from build123d import *

# Parameters (mm, degrees)
BOSS_EXTRUDE1_DEPTH            = 2
BOSS_EXTRUDE2_DEPTH            = 17.5
BOSS_EXTRUDE2_DEPTH_BACK       = 17.5
SKETCH2_R                      = 1.7500000000000036
SKETCH3_R                      = 2.999999999999994
CUT_EXTRUDE1_DEPTH             = 6.75
CUT_EXTRUDE2_DEPTH             = 2
BOSS_EXTRUDE4_DEPTH            = 3
BOSS_EXTRUDE4_DEPTH_BACK       = 0.5
SKETCH6_R                      = 1.7500000000000036
CUT_EXTRUDE3_DEPTH             = 77.9415362466854
FILLET1_R                      = 1
SKETCH7_W                      = 9
SKETCH7_H                      = 6
CUT_EXTRUDE4_DEPTH             = 2
FILLET2_R                      = 3
FILLET3_R                      = 3
CUT_EXTRUDE5_REACH             = 78.455
SKETCH10_R                     = 2.999999999999994
CUT_EXTRUDE5_DIRECTION_2_REACH = 78.455
BOSS_EXTRUDE6_DEPTH            = 1
BOSS_EXTRUDE6_DEPTH_BACK       = 1
SKETCH11_R                     = 0.7499999999999987
FILLET5_R                      = 1.5


# Some blends are built 0.0001 mm under size
with BuildPart() as part:
    # Sketch1 → Boss-Extrude1 (new body)
    with BuildSketch(Plane(origin=(0, 0, 0), x_dir=(1, 0, 0), z_dir=(0, 1, 0))):
        with BuildLine():
            Line((-17.499999999999993, -42), (17.499999999999993, -42))
            ThreePointArc((17.499999999999993, -42), (45.5, 1.01e-14), (17.499999999999975, 42.00000000000001))
            Line((17.499999999999975, 42.00000000000001), (-17.499999999999975, 42.00000000000001))
            ThreePointArc((-17.499999999999975, 42.00000000000001), (-45.5, 5.57e-15), (-17.499999999999993, -42))
        make_face()
    extrude(amount=BOSS_EXTRUDE1_DEPTH)

    # Sketch2 → Boss-Extrude2 (add, two sides: drawn at the far end of the back side and taken through both)
    with BuildSketch(Plane(origin=(0, 0, 0), x_dir=(0, 0, -1), z_dir=(1, 0, 0)).offset(-BOSS_EXTRUDE2_DEPTH_BACK)):
        with BuildLine():
            Line((-42, 0), (-42.171572875253815, 0))
            ThreePointArc((-42.171572875253815, 0), (-48.00000000000001, 1.0000000000000004), (-42.171572875253815, 2))
            Line((-42.171572875253815, 2), (-42, 2))
            Line((-42, 2), (-42, 1))
            Line((-42, 1), (-42, 0))
        make_face()
        with Locations((-45.00000000000001, 1)):
            Circle(SKETCH2_R, mode=Mode.SUBTRACT)
    extrude(amount=BOSS_EXTRUDE2_DEPTH + BOSS_EXTRUDE2_DEPTH_BACK)

    # Sketch3 → Cut-Extrude1 (cut)
    with BuildSketch(Plane(origin=(3.5, 0, 0), x_dir=(0, 0, -1), z_dir=(1, 0, 0))):
        with Locations((-45.00000000000001, 1)):
            Circle(SKETCH3_R)
    cut_extrude1 = extrude(amount=CUT_EXTRUDE1_DEPTH, mode=Mode.SUBTRACT)

    # Mirror1: Cut-Extrude1 across plane
    add(cut_extrude1.mirror(Plane(origin=(0, 0, 0), x_dir=(0, 0, 1), z_dir=(1, 0, 0))), mode=Mode.SUBTRACT)

    # Sketch4 → Cut-Extrude2 (cut)
    with BuildSketch(Plane(origin=(0, 2, 0), x_dir=(1, 0, 0), z_dir=(0, 1, 0))):
        Polygon((0.7499999999999764, 42.00000000000001), (21.249999999999982, 42.00000000000001), (21.24999999999998, 32.75000000000001), (0.7499999999999775, 32.75000000000001), (0.7499999999999781, 35.00000000000001), (-17.50000000000002, 35.00000000000001), (-17.50000000000002, 42.00000000000001), align=None)
    extrude(amount=-CUT_EXTRUDE2_DEPTH, mode=Mode.SUBTRACT)

    # Sketch5 → Boss-Extrude4 (add, two sides: drawn at the far end of the back side and taken through both)
    with BuildSketch(Plane(origin=(-17.50000000000002, 0, 0), x_dir=(0, 0, -1), z_dir=(1, 0, 0)).offset(-BOSS_EXTRUDE4_DEPTH_BACK)):
        with BuildLine():
            Line((35.00000000000001, 1), (35.00000000000001, 2))
            Line((35.00000000000001, 2), (38.171572875253815, 2))
            ThreePointArc((38.171572875253815, 2), (44.00000000000001, 1), (38.171572875253815, 0))
            Line((38.171572875253815, 0), (35.00000000000001, 0))
            Line((35.00000000000001, 0), (35.00000000000001, 1))
        make_face()
    extrude(amount=BOSS_EXTRUDE4_DEPTH + BOSS_EXTRUDE4_DEPTH_BACK)

    # Sketch6 → Cut-Extrude3 (cut, through all)
    with BuildSketch(Plane(origin=(-14.500000000000023, 0, 0), x_dir=(0, 0, -1), z_dir=(1, 0, 0))):
        with Locations((41.00000000000001, 1)):
            Circle(SKETCH6_R)
    extrude(amount=-CUT_EXTRUDE3_DEPTH, mode=Mode.SUBTRACT)

    # Fillet1
    fillet1_edges = [part.edges().sort_by_distance(p)[0] for p in [
        (-20.23555777714238, 0, -39.563859338365496),
        (-20.23555777714238, 2, -39.563859338365496),
    ]]
    fillet(fillet1_edges, radius=FILLET1_R - 0.0001)  # a hair under: the kernel refuses the full size

    # Sketch7 → Cut-Extrude4 (cut)
    with BuildSketch(Plane(origin=(0, 2, 0), x_dir=(1, 0, 0), z_dir=(0, 1, 0))):
        with Locations((24.749999999999975, 38.00000000000001)):
            Rectangle(SKETCH7_W, SKETCH7_H)
    extrude(amount=-CUT_EXTRUDE4_DEPTH, mode=Mode.SUBTRACT)

    # Fillet2
    # the kernel refuses this fillet: 3 mm, written as the material it adds along each edge
    with BuildSketch(Plane(origin=(-14.500000000000021, 0, -35.00000000000001), x_dir=(0, 0, -1), z_dir=(0, 1, 0))) as fillet2_piece_1:
        with BuildLine():
            CenterArc((FILLET2_R, -FILLET2_R), FILLET2_R, 90, 90)
            Line((0, -FILLET2_R), (0, 0))
            Line((0, 0), (FILLET2_R, 0))
        make_face()
    extrude(amount=2)
    # the kernel refuses this fillet: 3 mm, written as the material it takes off along each edge
    with BuildSketch(Plane(origin=(29.07318352021326, 4.856917413714078, -35.00000000000001), x_dir=(-1, 0, 0), z_dir=(0, -1, 0))) as fillet2_2_piece_1:
        with BuildLine():
            CenterArc((1.1044509783192602, -3), FILLET2_R, 90, 41.154201960072044)
            ThreePointArc((-0.8698124952261921, -0.7411764705882291), (-0.43723324041952694, -0.3678573776648406), (0, 0))
            Line((0, 0), (1.1044509783192602, 0))
        make_face()
    extrude(amount=7.7138348274281565, mode=Mode.SUBTRACT)
    with BuildSketch(Plane(origin=(21.24999999999998, -7.261843774138903, -35.00000000000001), x_dir=(0, 0, 1), z_dir=(0, 1, 0))) as fillet2_2_piece_2:
        with BuildLine():
            CenterArc((3, 2.904737509655561), FILLET2_R, 180, 75.52248781407008)
            Line((0, 2.904737509655561), (0, 0))
            Line((0, 0), (2.25, 0))
        make_face()
    extrude(amount=16.523687548277806, mode=Mode.SUBTRACT)
    with BuildSketch(Plane(origin=(0.7499999999999781, 9.261843774138908, -35.00000000000001), x_dir=(-1, 0, 0), z_dir=(0, -1, 0))) as fillet2_2_piece_3:
        with BuildLine():
            CenterArc((2.9047375096555634, -3), FILLET2_R, 90, 75.5224878140701)
            Line((7.8e-16, -2.25), (0, 0))
            Line((0, 0), (2.9047375096555634, 0))
        make_face()
    extrude(amount=16.523687548277817, mode=Mode.SUBTRACT)

    # Fillet3
    fillet3_edges = [part.edges().sort_by_distance(p)[0] for p in [
        (21.24999999999998, 1, -32.75000000000001),
        (0.7499999999999775, 1, -32.75000000000001),
    ]]
    fillet(fillet3_edges, radius=FILLET3_R)

    # Cut-Extrude5: up to this face of the body (flat: up to its plane)
    cut_extrude5_end = Plane(part.part.faces().sort_by_distance((-10.25, 1, 42.084852814))[0])
    # Sketch10 → Cut-Extrude5 (cut, up to the picked face)
    with BuildSketch(Plane.ZY.offset(13.874999999999995), mode=Mode.PRIVATE) as cut_extrude5_sk1:
        with Locations((45.00000000000001, 1)):
            Circle(SKETCH10_R)
    cut_extrude5_tool1 = split(extrude(cut_extrude5_sk1.sketch, amount=-CUT_EXTRUDE5_REACH, mode=Mode.PRIVATE), bisect_by=cut_extrude5_end, keep=Keep.BOTH, mode=Mode.PRIVATE)
    add(cut_extrude5_tool1.solids().sort_by(Axis((-13.875, 1, 45), (1, 0, 0)))[0], mode=Mode.SUBTRACT)

    # Cut-Extrude5 direction 2: up to this face of the body (flat: up to its plane)
    cut_extrude5_direction_2_end = Plane(part.part.faces().sort_by_distance((-17.5, 1.915147186, 42.085786438))[0])
    # Sketch10 → Cut-Extrude5 direction 2 (cut, up to the picked face)
    with BuildSketch(Plane.ZY.offset(13.874999999999995), mode=Mode.PRIVATE) as cut_extrude5_direction_2_sk1:
        with Locations((45.00000000000001, 1)):
            Circle(SKETCH10_R)
    cut_extrude5_direction_2_tool1 = split(extrude(cut_extrude5_direction_2_sk1.sketch, amount=CUT_EXTRUDE5_DIRECTION_2_REACH, mode=Mode.PRIVATE), bisect_by=cut_extrude5_direction_2_end, keep=Keep.BOTH, mode=Mode.PRIVATE)
    add(cut_extrude5_direction_2_tool1.solids().sort_by(Axis((-13.875, 1, 45), (-1, 0, 0)))[0], mode=Mode.SUBTRACT)

    # Sketch11 → Boss-Extrude6 (add, two sides: drawn at the far end of the back side and taken through both)
    with BuildSketch(Plane.ZY.offset(13.874999999999995).offset(-BOSS_EXTRUDE6_DEPTH_BACK)):
        Polygon((38.171572875253815, 2), (45.24264068711927, 9.07106781186549), (47.242640687119284, 7.071067811865485), (42.171572875253815, 2), align=None)
        with Locations((45.18198051533946, 7.010407640085664)):
            Circle(SKETCH11_R, mode=Mode.SUBTRACT)
    extrude(amount=BOSS_EXTRUDE6_DEPTH + BOSS_EXTRUDE6_DEPTH_BACK)

    # Fillet5
    # the kernel refuses this fillet: 1.5 mm, written as the material it adds along each edge
    with BuildSketch(Plane(origin=(-12.874999999999995, 2, 42.171572875253815), x_dir=(0, -0.9701770324837726, -0.24239745386653885), z_dir=(-1, 0, 0))) as fillet5_piece_1:
        with BuildLine():
            CenterArc((0.42686024849732124, 1.4932362441747078), FILLET5_R, 239.02808334302642, 36.41505394843642)
            Line((-0.3450665643766781, 0.2071067811865567), (0, 0))
            ThreePointArc((0, 0), (0.284573498998202, -0.01352751165058759), (0.5691469979964033, 2e-17))
        make_face()
    extrude(amount=2)
    with BuildSketch(Plane(origin=(-12.874999999999995, 2, 38.171572875253815), x_dir=(0, 0, -1), z_dir=(-1, 0, 0))) as fillet5_piece_2:
        with BuildLine():
            CenterArc((FILLET5_R * 0.414213562373, -FILLET5_R), FILLET5_R, 90, 45.000000000000085)
            Line((-FILLET5_R * 0.292893218813, -FILLET5_R * 0.292893218813), (0, 0))
            Line((0, 0), (FILLET5_R * 0.414213562373, 0))
        make_face()
    extrude(amount=2)
    # the kernel refuses this fillet: 1.5 mm, written as the material it takes off along each edge
    with BuildSketch(Plane(origin=(-18.625000000000014, 7.071067811865485, 47.242640687119284), x_dir=(0, 0.7071067811865455, -0.7071067811865496), z_dir=(1, 0, 0))) as fillet5_2_piece_1:
        with BuildLine():
            CenterArc((FILLET5_R, -FILLET5_R), FILLET5_R, 89.9999999999999, 90.00000000000017)
            Line((4.98e-15, -FILLET5_R), (0, 0))
            Line((0, 0), (FILLET5_R, 2e-17))
        make_face()
    extrude(amount=9.500000000000039, mode=Mode.SUBTRACT)
    with BuildSketch(Plane(origin=(-18.62499999999999, 9.07106781186549, 45.24264068711927), x_dir=(0, -0.7071067811865499, -0.7071067811865451), z_dir=(1, 0, 0))) as fillet5_2_piece_2:
        with BuildLine():
            CenterArc((FILLET5_R, -FILLET5_R), FILLET5_R, 90.0000000000001, 89.99999999999984)
            Line((1.28e-15, -FILLET5_R), (0, 0))
            Line((0, 0), (FILLET5_R, 9e-17))
        make_face()
    extrude(amount=9.49999999999999, mode=Mode.SUBTRACT)


solid = part.part
Work out the finished part from the listing and answer in its coordinate system (mm). A direction names the side the tool comes from. Give positions to 0.01 mm unless a question says otherwise; leave off trailing zeros. Order: outer loops, then holes, each group sorted by start corner. A loop starts at its lowest first (then second) coordinate and runs counter-clockwise, first axis right, second up. Notation, with made-up numbers: (-17, -30.75) -> (19, -30.75) arc R36 ccw to (19, 7.25) -> close; hole circle Ø4 at (21, 57). An arc over 180 degrees is marked (long way). Answer as a JSON object with one key per item and string values. Group by question number.
1. Section C-C on z = 35.5 is taken. Determine the outline of the cut face in (x, y).
2. Section B-B on z = -17 is taken. Determine the outline of the cut face in (x, y), plus the area to 3 significant figures.
3. A tool of negligible diameter and unlimited length cuts with its end or side. For faces 1 (the cylindrical face through (-16, 1, -44)), 2 (the flat face through (-7, 1, -35)), from which of +Z, -Z, +X, -X, +Y, -Y can it reach the whole face along a straight path? Write none if from no direction.
4. Consider line 1 along Y through (x, z) = (-17.75, -41); line 2 along Y through (x, z) = (9, -1); line 3 along X through (y, z) = (1.5, -33). Determine where each line is inside the solid, lowest interval first. Write a range as [from, to].
5. Flat-ended cylindrical pins translate along their axes: pin 1 Ø5 at (y, z) = (2, 45) entering from -X (3 decimals); pin 2 Ø5.5 at (y, z) = (6.5, 40.5) entering from +X (3 decimals); pin 3 Ø5 at (x, z) = (16.5, 9) entering from +Y; pin 4 Ø0.9 at (y, z) = (7.01, 45.18) entering from -X. Find the tip coordinate at first contact, or state that the pin passes through.
6. Section A-A on z = -41 is taken. Determine the outline of the cut face in (x, y), plus the area to 3 significant figures.
7. The mould has two halves that part along Y. Classify faces 3 (the cylindrical face through (14, 1, 48)), 4 (the cylindrical face through (-16.81, 1.08, -39.25)), 5 (the flat face through (-1, 2, 1)), 6 (the flat face through (-14.5, 1, -39)): released by +Y, released by -Y, zero draft, split by the parting line, or undercut.
Result sheet:
{
 "1": {"outline": "(-28.46, 0) -> (28.46, 0) -> (28.46, 2) -> (-28.46, 2) -> close"},
 "2": {"outline": "(-42.2, 0) -> (42.2, 0) -> (42.2, 2) -> (-42.2, 2) -> close", "area": "169 mm^2"},
 "3": {"face 1": "+X, -X", "face 2": "-Z, +X, +Y, -Y"},
 "4": {"line 1": "y = [-2, -0.75], [2.75, 4]", "line 2": "y = [0, 2]", "line 3": "x = [-31.32, 1.33], [20.67, 31.32]"},
 "5": {"pin 1": "stops at x = -14.875", "pin 2": "stops at x = -12.875", "pin 3": "stops at y = 2", "pin 4": "passes through"},
 "6": {"outline": "(-18, -2) -> (-14.5, -2) -> (-14.5, -0.75) -> (-18, -0.75) -> close; (-18, 2.75) -> (-14.5, 2.75) -> (-14.5, 4) -> (-18, 4) -> close", "area": "8.75 mm^2"},
 "7": {"face 3": "split by the parting line", "face 4": "undercut", "face 5": "released by +Y", "face 6": "zero draft"}
}
